Read the model definition and answer for the solid it produces. Units are mm, in the model's axes. A direction names the side the tool comes from. Give positions to 0.01 mm unless a question says otherwise; leave off trailing zeros. Order: outer loops, then holes, each group sorted by start corner. A loop starts at its lowest first (then second) coordinate and runs counter-clockwise, first axis right, second up. Notation, with made-up numbers: (58.25, -38) -> (73.25, -38) arc R25 ccw to (73.25, -7) -> close; hole circle Ø10 at (54.5, -23.75). An arc over 180 degrees is marked (long way). Use one line per item in the form item = value.
```python
from build123d import *

# Parameters (mm, degrees)
F0_W     = 120
F0_H     = 63.066
F1_DEPTH = 3
F3_D     = 3
F4_W     = 3
F4_H     = 30
F5_DEPTH = 3.001


with BuildPart() as f1:
    # F0 (on Top) → F1 (new body)
    with BuildSketch(Plane.XY):
        Rectangle(F0_W, F0_H)
    extrude(amount=F1_DEPTH)

    # F3 (through all)
    with Locations(Plane.XY.offset(3)):
        with Locations((-48, 29.033), (48, 29.033), (48, -29.033), (-48, -29.033)):
            Hole(F3_D / 2)

    # F4 (on face) → F5 (cut, through all)
    with BuildSketch(Plane.XY.offset(3)):
        with Locations((-34.4999431167, 0)):
            Rectangle(F4_W, F4_H)
        with Locations((-24.4999431167, 0)):
            Rectangle(F4_W, F4_H)
        with Locations((-14.4999431167, 0)):
            Rectangle(F4_W, F4_H)
        with Locations((5.5000568833, 0)):
            Rectangle(F4_W, F4_H)
        with Locations((-4.4999431167, 0)):
            Rectangle(F4_W, F4_H)
        with Locations((15.5000568833, 0)):
            Rectangle(F4_W, F4_H)
        with Locations((25.5000568833, 0)):
            Rectangle(F4_W, F4_H)
        with Locations((35.5000568833, 0)):
            Rectangle(F4_W, F4_H)
    extrude(amount=-F5_DEPTH, mode=Mode.SUBTRACT)


solid = f1.part
```
Item 1: The part is cut by section B-B on y = -12.5. State how many separate pieces and enclosed holes the cut face has, and give its area (3 significant figures).
Checks:
separate_pieces = 9
enclosed_holes = 0
area = 288 mm²
Item 2: Given pin 1 Ø5 at (x, y) = (-48, 29.033) entering from +Z; pin 2 Ø2.5 at (x, y) = (48, -29.033) entering from -Z, each flat-ended and moving along its own axis, determine where each tip first touches the part or whether it passes through.
Checks:
pin_1 = 3
pin_2 = through
Item 3: The part is cut by section A-A on x = 48. Give the vertices of the cut face in (y, z).
Checks:
outline = (-31.53, 0) -> (-30.53, 0) -> (-30.53, 3) -> (-31.53, 3) -> close; (-27.53, 0) -> (27.53, 0) -> (27.53, 3) -> (-27.53, 3) -> close; (30.53, 0) -> (31.53, 0) -> (31.53, 3) -> (30.53, 3) -> close
Item 4: Determine the mould class of faces 1 (the cylindrical face through (-46.81, 28.12, 1.48)), 2 (the flat face through (-1, 31.533, 1)) for opening direction X: +X half, -X half, draft (parallel to the pull), parting line (faces both ways), or undercut.
Checks:
face_1 = undercut
face_2 = draft
Item 5: Which of the six approach directions +Z, -Z, +X, -X, +Y, -Y give full straight-line access (tool end or side, diameter ignored) to faces 3 (the flat face through (-15, 15, 2)), 4 (the flat face through (-1, 0, 0))?
Checks:
face_3 = +Z, -Z
face_4 = -Z, +X, -X, +Y, -Y
Item 6: Straight lines are drawn through the part: L1, parallel to Y at x = -48, z = 1.05; L2, parallel to Y at x = 47, z = 2.7; L3, parallel to Y at x = 36.5, z = 1.55. For each, find the intervals that lie inside material, in ascending order. Write a range as from..to.
Checks:
L1 = -31.53..-30.53, -27.53..27.53, 30.53..31.53
L2 = -31.53..-30.15, -27.91..27.91, 30.15..31.53
L3 = -31.53..-15, 15..31.53
